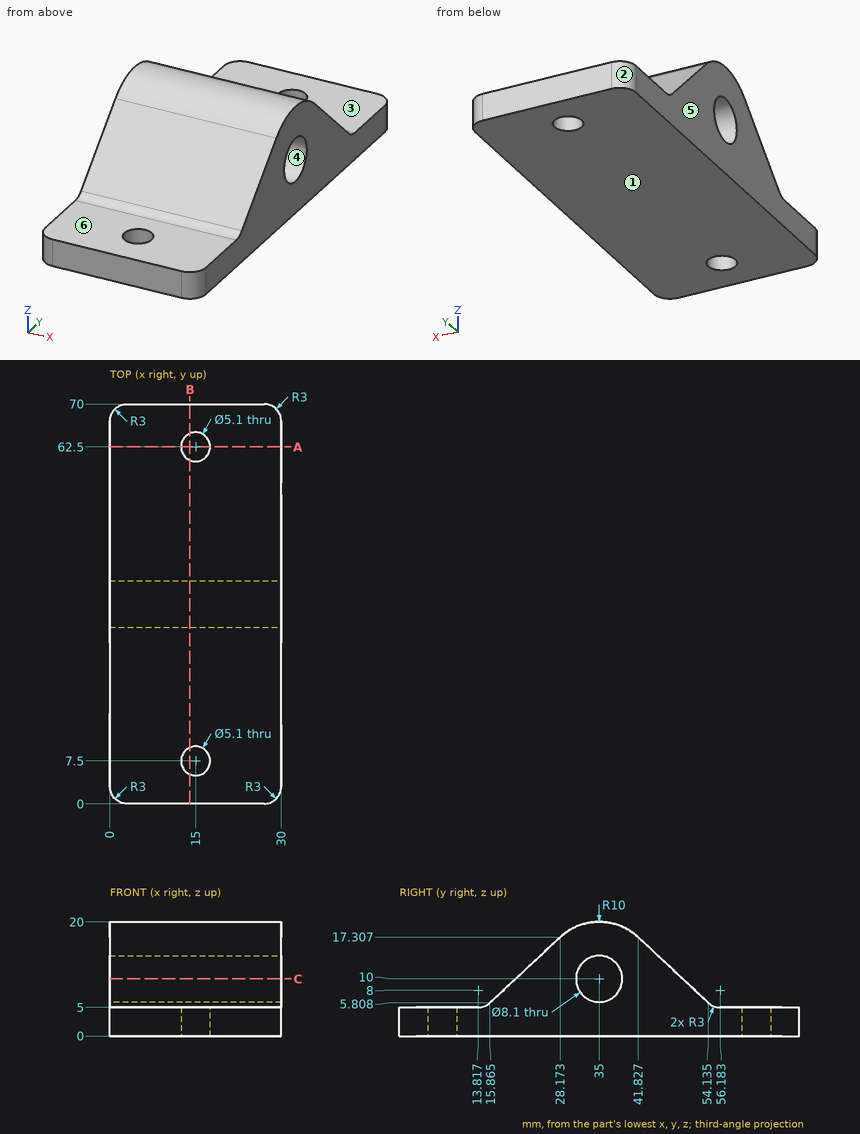
Design review of the part shown in the three views and the two pictorial views. Dimensions are in mm from the part's minimum x, y and z. A direction names the side the tool comes from. Give positions to 0.01 mm unless a question says otherwise; leave off trailing zeros. Loops run counter-clockwise (first coordinate to the right, second up) from the corner with the lowest first, then second, coordinate; pieces in that order, holes last. Notation, with made-up numbers: (-16, 37) - (-4, 37) arc R38 cw to (-4, 76) - close; hole circle Ø7 at (35.25, -32). An arc over 180 degrees is marked (long way). Answer as a JSON object with one key per item and string values.
Q1. Mouldability with a two-part tool opening along Z and no side actions: class the marked faces 1, 2, 3 and 4 as +Z half, -Z half, draft (parallel to the pull), parting line (faces both ways), or undercut.
Worked out:
{"face 1": "-Z half", "face 2": "draft", "face 3": "+Z half", "face 4": "undercut"}
Q2. Add section A-A on y = 62.5. State the section outline as (x, z) points, plus the area to 4 significant figures.
Worked out:
{"outline": "(0, 0) - (12.45, 0) - (12.45, 5) - (0, 5) - close; (17.55, 0) - (30, 0) - (30, 5) - (17.55, 5) - close", "area": "124.5 mm^2"}
Q3. Add section B-B on x = 14. Count the separate pieces of the cut face and the enclosed holes in it, plus the area to 3 significant figures.
Worked out:
{"separate pieces": "3", "enclosed holes": "1", "area": "607 mm^2"}
Q4. Add section C-C on z = 10. State the section outline as (x, y) points, plus the area to 3 significant figures.
Worked out:
{"outline": "(0, 20.35) - (30, 20.35) - (30, 30.95) - (0, 30.95) - close; (0, 39.05) - (30, 39.05) - (30, 49.65) - (0, 49.65) - close", "area": "636 mm^2"}
Q5. To check wall thickness, follow line 1 along Y through (x, z) = (15, 2.7); line 2 along Z through (x, y) = (23, 4); line 3 along Z through (x, y) = (26.25, 37). State the ranges of each line that lie inside material, in increasing order.
Worked out:
{"line 1": "y = 0 to 4.95, 10.05 to 59.95, 65.05 to 70", "line 2": "z = 0 to 5", "line 3": "z = 0 to 6.48, 13.52 to 19.8"}
Q6. Insertion check: pin 1 (11 mm diameter, centred on x = 19, y = 5.5, fed in from +Z); pin 2 (8 mm diameter, centred on x = 12.5, z = 18, fed in from -Y); pin 3 (3 mm diameter, centred on x = 15, y = 7.5, fed in from -Z); pin 4 (1 mm diameter, centred on x = 7.5, z = 12.5, fed in from +Y). Each pin has a flat end and moves straight along its axis. Give the tip position at first contact, or say it passes through.
Worked out:
{"pin 1": "stops at z = 5", "pin 2": "stops at y = 24.63", "pin 3": "passes through", "pin 4": "stops at y = 47.51"}
Q7. For the marked faces 5 and 6, list the 3-axis set-ups (+Z, -Z, +X, -X, +Y, -Y) from which the entire face can be reached by the end or side of a thin tool; tool diameter is ignored.
Worked out:
{"face 5": "+Z, -Z, -X, +Y, -Y", "face 6": "+Z, +X, -X, -Y"}
